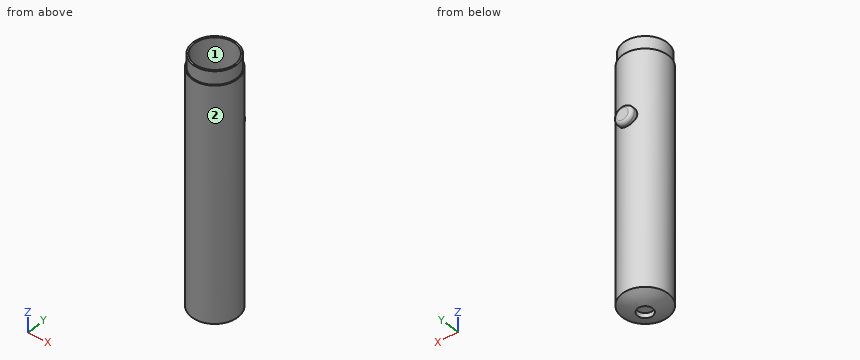
Autodesk Inventor part; units mm, degrees
ref_plane "YZ Plane" through (0, 0, 0) normal (1, 0, 0) x (0, 1, 0)
ref_plane "XZ Plane" through (0, 0, 0) normal (0, 1, 0) x (-1, 0, 0)
ref_plane "XY Plane" through (0, 0, 0) normal (0, 0, 1) x (1, 0, 0)
sketch "Sketch1" plane through (0, 0, 0) normal (1, 0, 0) x (0, 1, 0)
  line L0 (0, 0) -> (6.1, 0) construction
  line L1 (6.6, 0) -> (6.6, -4)
  line L2 (6.6, -4) -> (6.95, -4)
  line L3 (6.95, -4) -> (6.95, -74.9)
  line L4 (6.95, -74.9) -> (0, -74.9) construction
  line L5 (0, -74.9) -> (0, -15)
  arc A0 (2.25, -76.9) -> (6.95, -74.9) centre (0, -65.09) ccw
  line L6 (2.25, -76.9) -> (2.25, -75.4)
  line L7 (2.25, -75.4) -> (0, -75.4)
  line L8 (0, -75.4) -> (0, -74.9)
  line L9 (6.1, 0) -> (6.1, -15)
  line L10 (6.1, -15) -> (0, -15)
  line L11 (6.1, 0) -> (6.6, 0)
  line L12 (0, -15) -> (0, 0) construction
  dimension "d0" = 6.95
  dimension "d1" = 6.6
  dimension "d2" = 4
  dimension "d4" = 76.9
  dimension "d5" = 2.25
  dimension "d6" = 1.5
  dimension "d7" = 2
  dimension "d9" = 0.5
  dimension "d10" = 15
revolve "Revolution1" add sketch "Sketch1" angle 360 about axis through (0, 0, -74.9) along (0, 0, 1)
sketch "Sketch2" plane through (0, 0, 0) normal (0, 1, 0) x (-1, 0, 0)
  line L0 (0, 0) -> (0, -26)
  line L1 (0, -26) -> (16.769, -26) construction
  circle A0 centre (0, -23.25) radius 2.75
  line L2 (-6.6, 0) -> (6.6, 0)
  dimension "d12" = 5.5
  dimension "d11" = 26
extrude "Extrusion1" add sketch "Sketch2" along normal blind 8.5
fillet "Fillet1" radius 1 1 edges at (2.75, 8.5, -23.25)
properties part number "LASER"
Source: CAD feature listing. Evaluate the final solid. Frame: model axes, mm. Face numbers are marked on the shaded views. Coordinates: 2 decimals unless noted, no trailing zeros. Loops run counter-clockwise (first coordinate to the right, second up) from the corner with the lowest first, then second, coordinate; pieces in that order, holes last. Notation, with made-up numbers: M 17,82.5 L 23,82.5 A22 ccw 23,108.5 Z; hole C 24,73.5 d10. An arc over 180 degrees is marked long. Use a Markdown table: item, result. Add a question column.
Q1. First-contact query: pin 1 (5 mm diameter, centred on x = 4, z = -39.5, fed in from +Y); pin 2 (8 mm diameter, centred on x = 4.5, z = -10, fed in from +Y); pin 3 (3.5 mm diameter, centred on x = 0, y = 0, fed in from +Z). Flat tips, straight axial feed; report the tip coordinate or a pass-through.
Q2. Section query A-A, the plane x = 0. Return loops of the section in (y, z).
Q3. Section query B-B, the plane y = 0. Return loops of the section in (x, z), and give its area (3 significant figures).
Q4. Material intervals for L1, parallel to Y at x = 0, z = -10.5; L2, parallel to X at y = 0, z = -76.1, sorted ascending.
Q5. Section query D-D, the plane y = 5. Return loops of the section in (x, z), and give its area (3 significant figures).
Q6. Draft query along Y for the marked faces 1 and 2. Return one class per face: pulls with the +Y half, pulls with the -Y half, needs draft (parallel to the pull), parting line crosses it, or undercut.
Q7. Section query C-C, the plane z = -23.25. Return loops of the section in (x, y), and give its area (3 significant figures).
Result:
| question | item | result |
|---|---|---|
| 1 | pin 1 | stops at y = 6.79 |
| 1 | pin 2 | stops at y = 6.93 |
| 1 | pin 3 | stops at z = -15 |
| 2 | outline | M -6.95,-74.9 A12.02 ccw -2.25,-76.9 L -2.25,-75.4 L 2.25,-75.4 L 2.25,-76.9 A12.02 ccw 6.95,-74.9 L 6.95,-26 L 7.5,-26 A1 ccw 8.5,-25 L 8.5,-21.5 A1 ccw 7.5,-20.5 L 6.95,-20.5 L 6.95,-4 L 6.6,-4 L 6.6,0 L 6.1,0 L 6.1,-15 L -6.1,-15 L -6.1,0 L -6.6,0 L -6.6,-4 L -6.95,-4 Z |
| 3 | outline | M -6.95,-74.9 A12.02 ccw -2.25,-76.9 L -2.25,-75.4 L 2.25,-75.4 L 2.25,-76.9 A12.02 ccw 6.95,-74.9 L 6.95,-4 L 6.6,-4 L 6.6,0 L 6.1,0 L 6.1,-15 L -6.1,-15 L -6.1,0 L -6.6,0 L -6.6,-4 L -6.95,-4 Z |
| 3 | area | 869 mm2 |
| 4 | L1 | y = -6.95 to -6.1, 6.1 to 6.95 |
| 4 | L2 | x = -4.83 to -2.25, 2.25 to 4.83 |
| 5 | outline | M -4.83,-74.9 A10.93 ccw 4.83,-74.9 L 4.83,-4 L 4.31,-4 L 4.31,0 L 3.49,0 L 3.49,-15 L -3.49,-15 L -3.49,0 L -4.31,0 L -4.31,-4 L -4.83,-4 Z |
| 5 | area | 621 mm2 |
| 6 | face 1 | undercut |
| 6 | face 2 | parting line crosses it |
| 7 | outline | M -2.75,6.38 A6.95 ccw long 2.75,6.38 L 2.75,7.5 A1 ccw 1.75,8.5 L -1.75,8.5 A1 ccw -2.75,7.5 Z |
| 7 | area | 161 mm2 |
